from build123d import *

# Parameters (mm, degrees)
SKETCH1_W           = 178.16
SKETCH1_H           = 120
BOSS_EXTRUDE1_DEPTH = 3
SKETCH2_R           = 14.225
SKETCH2_R_2         = 2.75
SKETCH2_R_3         = 3.375
CUT_EXTRUDE1_DEPTH  = 4
SKETCH3_R           = 2.0193
CUT_EXTRUDE2_DEPTH  = 4
SKETCH6_R           = 2.5
CUT_EXTRUDE3_DEPTH  = 4
SKETCH7_W           = 16.5
SKETCH7_H           = 45
CUT_EXTRUDE4_DEPTH  = 4


with BuildPart() as part:
    # Sketch1 → Boss-Extrude1 (new body)
    with BuildSketch(Plane.XY):
        with Locations((89.08, -60)):
            Rectangle(SKETCH1_W, SKETCH1_H)
    extrude(amount=BOSS_EXTRUDE1_DEPTH)

    # Sketch2 → Cut-Extrude1 (cut, through all)
    with BuildSketch(Plane.XY.offset(3)):
        with Locations((26.5, -35)):
            Circle(SKETCH2_R)
        with Locations((151.66, -35)):
            Circle(SKETCH2_R)
        with Locations((26.5, -110)):
            Circle(SKETCH2_R_2)
        with Locations((151.66, -110)):
            Circle(SKETCH2_R_2)
        with Locations((89.08, -8)):
            Circle(SKETCH2_R_3)
        with Locations((26.5, -95)):
            Circle(SKETCH2_R_2)
        with Locations((151.66, -95)):
            Circle(SKETCH2_R_2)
    extrude(amount=-CUT_EXTRUDE1_DEPTH, mode=Mode.SUBTRACT)

    # Sketch3 → Cut-Extrude2 (cut, through all)
    with BuildSketch(Plane(origin=(0, 0, 0), x_dir=(-1, 0, 0), z_dir=(0, 0, -1))):
        with Locations((-44.460512242, -52.960512242)):
            Circle(SKETCH3_R)
        with Locations((-26.5, -9.6)):
            Circle(SKETCH3_R)
        with Locations((-8.539487758, -17.039487758)):
            Circle(SKETCH3_R)
        with Locations((-26.5, -60.4)):
            Circle(SKETCH3_R)
        with Locations((-133.699487758, -17.039487758)):
            Circle(SKETCH3_R)
        with Locations((-151.66, -9.6)):
            Circle(SKETCH3_R)
        with Locations((-151.66, -60.4)):
            Circle(SKETCH3_R)
        with Locations((-169.620512242, -52.960512242)):
            Circle(SKETCH3_R)
    extrude(amount=-CUT_EXTRUDE2_DEPTH, mode=Mode.SUBTRACT)

    # Sketch6 → Cut-Extrude3 (cut, through all)
    with BuildSketch(Plane.XY.offset(3)):
        with Locations((26.5, -60.4)):
            Circle(SKETCH6_R)
        with Locations((44.460512242, -52.960512242)):
            Circle(SKETCH6_R)
        with Locations((26.5, -9.6)):
            Circle(SKETCH6_R)
        with Locations((8.539487758, -17.039487758)):
            Circle(SKETCH6_R)
        with Locations((169.620512242, -52.960512242)):
            Circle(SKETCH6_R)
        with Locations((151.66, -60.4)):
            Circle(SKETCH6_R)
        with Locations((133.699487758, -17.039487758)):
            Circle(SKETCH6_R)
        with Locations((151.66, -9.6)):
            Circle(SKETCH6_R)
    extrude(amount=-CUT_EXTRUDE3_DEPTH, mode=Mode.SUBTRACT)

    # Sketch7 → Cut-Extrude4 (cut, through all)
    with BuildSketch(Plane.XY.offset(3)):
        with Locations((169.91, -97.5)):
            Rectangle(SKETCH7_W, SKETCH7_H)
        with Locations((8.25, -97.5)):
            Rectangle(SKETCH7_W, SKETCH7_H)
    extrude(amount=-CUT_EXTRUDE4_DEPTH, mode=Mode.SUBTRACT)


solid = part.part
Read the model definition and answer for the solid it produces. Units are mm, in the model's axes. Coordinates: 2 decimals unless noted, no trailing zeros. Write each loop counter-clockwise with the first axis right and the second up, starting at its lowest first coordinate (ties: lowest second). Pieces come first, ordered by that corner, then holes. Notation, with made-up numbers: M 63,30 L 74,30 A18 cw 74,38 Z; hole C 68.25,50.25 d9. An arc over 180 degrees is marked long. Use a Markdown table: item, result.
Q1. The part is cut by section A-A, the plane y = -110. Write down the section's boundary in (x, z).
Answer block:
| item | result |
|---|---|
| outline | M 16.5,0 L 23.75,0 L 23.75,3 L 16.5,3 Z; M 29.25,0 L 148.91,0 L 148.91,3 L 29.25,3 Z; M 154.41,0 L 161.66,0 L 161.66,3 L 154.41,3 Z |
Q2. Straight lines are drawn through the part: L1, parallel to Y at x = 26.5, z = 0.75 (3 decimals); L2, parallel to X at y = -19, z = 0.6; L3, parallel to X at y = -61, z = 2.05. For each, find the intervals that lie inside material, in ascending order. Write a range as [from, to].
Answer block:
| item | result |
|---|---|
| L1 | y = [-120, -112.75], [-107.25, -97.75], [-92.25, -62.9], [-57.9, -49.225], [-20.775, -12.1], [-7.1, 0] |
| L2 | x = [0, 6.99], [10.09, 132.15], [135.25, 178.16] |
| L3 | x = [0, 24.07], [28.93, 149.23], [154.09, 178.16] |
Q3. Determine the mould class of faces 1 (the face through (85.71, -7.85, 1.52)), 2 (the face through (88, -59, 0)) for opening direction X: released by +X, released by -X, zero draft, split by the parting line, or undercut.
Answer block:
| item | result |
|---|---|
| face 1 | undercut |
| face 2 | zero draft |
Q4. The part is cut by section C-C, the plane z = 2.15. Give the number of separate pieces and of enclosed holes in the cut face, then the cut area to 3 significant figures.
Answer block:
| item | result |
|---|---|
| separate pieces | 1 |
| enclosed holes | 15 |
| area | 18,300 mm2 |
Q5. Each of these flat-tipped pins is pushed along its axis until it touches: pin 1 Ø3.5 at (x, y) = (26.5, -95) entering from -Z; pin 2 Ø1.5 at (y, z) = (-91, 1.5) entering from +X; pin 3 Ø1.5 at (x, z) = (167.5, 1.5) entering from -Y. Where does it stop, or does it pass through?
Answer block:
| item | result |
|---|---|
| pin 1 | passes through |
| pin 2 | stops at x = 161.66 |
| pin 3 | stops at y = -75 |
Q6. The part is cut by section B-B, the plane x = 89.08. Write down the section's boundary in (y, z) (3 decimals), then the cut area to 3 significant figures.
Answer block:
| item | result |
|---|---|
| outline | M -120,0 L -11.375,0 L -11.375,3 L -120,3 Z; M -4.625,0 L 0,0 L 0,3 L -4.625,3 Z |
| area | 340 mm2 |
Q7. The part is cut by section D-D, the plane y = -60.4. Write down the section's boundary in (x, z).
Answer block:
| item | result |
|---|---|
| outline | M 0,0 L 24,0 L 24,3 L 0,3 Z; M 29,0 L 149.16,0 L 149.16,3 L 29,3 Z; M 154.16,0 L 178.16,0 L 178.16,3 L 154.16,3 Z |
